Autodesk Inventor part; units mm, degrees
ref_plane "YZ Plane" through (0, 0, 0) normal (1, 0, 0) x (0, 1, 0)
ref_plane "XZ Plane" through (0, 0, 0) normal (0, 1, 0) x (-1, 0, 0)
ref_plane "XY Plane" through (0, 0, 0) normal (0, 0, 1) x (1, 0, 0)
sketch "Sketch1" plane through (0, 0, 0) normal (0, 0, 1) x (1, 0, 0)
  line L0 (0, 0) -> (-45.72, 0)
  line L1 (-45.72, 0) -> (-45.72, 20.32)
  line L2 (-45.72, 20.32) -> (0, 20.32)
  line L3 (0, 20.32) -> (0, 0)
  dimension "d0" = 45.72
  dimension "d1" = 20.32
extrude "Extrusion1" add sketch "Sketch1" along normal blind 4.826
sketch "Sketch2" plane through (-45.72, 0, 0) normal (0, -1, 0) x (1, 0, 0)
  line L0 (45.72, 0) -> (45.72, 4.826)
  line L1 (0, 0) -> (0, 4.826)
  line L2 (0, 0) -> (45.72, 0)
  line L3 (0, 4.826) -> (45.72, 4.826)
  line L4 (45.72, 0) -> (45.72, -28.194)
  line L5 (45.72, 4.826) -> (45.72, 20.066)
  line L6 (45.72, 20.066) -> (0, 20.066)
  line L7 (0, 20.066) -> (0, 4.826)
  line L8 (0, 0) -> (0, -28.194)
  line L9 (0, -28.194) -> (45.72, -28.194)
  line L10 (45.72, 0) -> (45.72, 4.826)
  line L11 (0, 4.826) -> (0, 0)
  dimension "d4" = 28.194
  dimension "d5" = 15.24
extrude "Extrusion2" add sketch "Sketch2" along normal blind 4.826
sketch "Sketch3" plane through (-45.72, 0, 0) normal (0, 1, 0) x (1, 0, 0)
  line L0 (45.72, 0) -> (0, 0)
  line L1 (45.72, 28.194) -> (45.72, 0)
  line L2 (0, 28.194) -> (45.72, 28.194)
  line L3 (0, 0) -> (0, 28.194)
  line L4 (22.86, 0) -> (22.86, 9.144) construction
  line L5 (22.86, 9.144) -> (45.72, 9.144)
  line L6 (22.86, 9.144) -> (0, 9.144)
  line L7 (45.72, 9.144) -> (45.72, 12.954)
  line L8 (45.72, 28.194) -> (45.72, -20.066)
  line L9 (45.72, 12.954) -> (0, 12.954)
  line L10 (0, 12.954) -> (0, 9.144)
  dimension "d8" = 9.144
  dimension "d9" = 3.81
extrude "Extrusion3" add sketch "Sketch3" along normal blind 20.32 contours L5 L6 L3 L9 L1
sketch "Sketch4" plane through (0, 0, -12.954) normal (0, 0, -1) x (-1, 0, 0)
  line L0 (0, 0) -> (0, 20.32)
  line L1 (0, 20.32) -> (45.72, 20.32)
  line L2 (45.72, 0) -> (45.72, 20.32)
  line L3 (45.72, 0) -> (0, 0)
  line L4 (22.86, 20.32) -> (22.86, 13.97) construction
  line L5 (22.86, 13.97) -> (30.48, 13.97) construction
  circle A0 centre (30.48, 13.97) radius 2.413
  circle A1 centre (15.24, 13.97) radius 2.413
  dimension "d12" = 6.35
  dimension "d13" = 7.62
  dimension "d14" = 4.826
extrude "Extrusion4" cut sketch "Sketch4" against normal through all contours A0 | A1
sketch "Sketch5" plane through (-45.72, 0, 0) normal (0, 1, 0) x (1, 0, 0)
  line L0 (45.72, 12.954) -> (0, 12.954)
  line L1 (0, 28.194) -> (45.72, 28.194)
  line L2 (45.72, 28.194) -> (45.72, 12.954) construction
  line L3 (0, 12.954) -> (0, 28.194)
  line L4 (45.72, 28.194) -> (45.72, -20.066)
  line L5 (45.72, 28.194) -> (45.72, 12.954) construction
  line L6 (45.72, 20.574) -> (0, 20.574) construction
  line L7 (22.86, 12.954) -> (22.86, 20.574) construction
  line L8 (22.86, 20.574) -> (13.97, 20.574) construction
  line L9 (22.86, 20.574) -> (31.75, 20.574) construction
  circle A0 centre (31.75, 20.574) radius 2.413
  circle A1 centre (13.97, 20.574) radius 2.413
  line L10 (45.72, 4.064) -> (0, 4.572) construction
  line L11 (0, 0) -> (0, 9.144)
  circle A2 centre (31.3866, -12.1315) radius 2.413
  circle A3 centre (13.611, -11.7365) radius 2.413
  point P0 (45.72, 0)
  dimension "d17" = 8.89
  dimension "d18" = 8.89
  dimension "d19" = 4.826
  dimension "d20" = 4.826
extrude "Extrusion5" cut sketch "Sketch5" against normal through all contours A0 | A1 | A2 | A3
properties part number "arm_to_tower_adapter"
Geometry check sheet. Reference: the model listing, model coordinates, mm. A direction names the side the tool comes from. Coordinates: 2 decimals unless noted, no trailing zeros. Order: outer loops, then holes, each group sorted by start corner. A loop starts at its lowest first (then second) coordinate and runs counter-clockwise, first axis right, second up. Notation, with made-up numbers: (-22, 83.5) -> (-7, 83.5) arc R18 cw to (-7, 92.5) -> close; hole circle Ø3 at (42.25, 27). An arc over 180 degrees is marked (long way). Use a Markdown table: item, result. Add a question column.
1. Cross-section at A-A (y = 1.75). Enter the section's corners in (x, z), and give its area (3 significant figures).
2. Set-up check for faces 4 (the face through (-23, 0, 13)), 5 (the face through (-23, 0, -20)), 6 (the face through (-12.83, 14.08, -11.08)), 7 (the face through (-23, -2, -28.194)), 8 (the face through (-23, 10, 0)): record each of +Z, -Z, +X, -X, +Y, -Y from which the full face is reachable in a straight line by a thin tool's end or side.
3. Cross-section at B-B (x = -31.75). Enter the section's corners in (y, z).
4. Cross-section at D-D (z = -10). Enter the section's corners in (x, y).
5. Cross-section at C-C (y = 13.97). Enter the section's corners in (x, z).
6. Go/stop test with flat-tipped pins: pin 1 Ø5 at (x, z) = (-26, -20.5) entering from +Y; pin 2 Ø10 at (x, y) = (-12.5, 12) entering from +Z; pin 3 Ø5.5 at (x, y) = (-15.24, 13.97) entering from -Z. Record where each tip stops, or that it passes through.
7. Material ranges on L1, parallel to Z at x = -43, y = 16.25; L2, parallel to Y at x = -15, z = 1; L3, parallel to X at y = 15, z = 2.5, recorded low to high.
8. Mould release check, pull along X, two halves, no side actions. Record for faces 1 (the face through (-23, 20.32, -11)), 2 (the face through (-14.856, -2.379, 14.487)), 3 (the face through (0, -0.5, -4.4)): pulls with the +X half, pulls with the -X half, needs draft (parallel to the pull), parting line crosses it, or undercut.
Filled sheet:
| question | item | result |
|---|---|---|
| 1 | outline | (-45.72, -12.95) -> (0, -12.95) -> (0, -9.14) -> (-45.72, -9.14) -> close; (-45.72, 0) -> (0, 0) -> (0, 4.83) -> (-45.72, 4.83) -> close |
| 1 | area | 395 mm2 |
| 2 | face 4 | +Z, +X, -X, +Y |
| 2 | face 5 | -Z, +X, -X, +Y |
| 2 | face 6 | +Z, -Z |
| 2 | face 7 | -Z, +X, -X, +Y, -Y |
| 2 | face 8 | +X, -X, +Y |
| 3 | outline | (-4.83, -28.19) -> (0, -28.19) -> (0, -22.99) -> (-4.83, -22.99) -> close; (-4.83, -18.16) -> (0, -18.16) -> (0, -12.95) -> (11.92, -12.95) -> (11.92, -9.14) -> (0, -9.14) -> (0, 0) -> (11.92, 0) -> (11.92, 4.83) -> (0, 4.83) -> (0, 9.35) -> (-4.83, 9.35) -> close; (-4.83, 14.12) -> (0, 14.12) -> (0, 20.07) -> (-4.83, 20.07) -> close; (16.02, -12.95) -> (20.32, -12.95) -> (20.32, -9.14) -> (16.02, -9.14) -> close; (16.02, 0) -> (20.32, 0) -> (20.32, 4.83) -> (16.02, 4.83) -> close |
| 4 | outline | (-45.72, -4.83) -> (0, -4.83) -> (0, 20.32) -> (-45.72, 20.32) -> close; hole circle Ø4.83 at (-30.48, 13.97); hole circle Ø4.83 at (-15.24, 13.97) |
| 5 | outline | (-45.72, -12.95) -> (-32.89, -12.95) -> (-32.89, -9.14) -> (-45.72, -9.14) -> close; (-45.72, 0) -> (-32.89, 0) -> (-32.89, 4.83) -> (-45.72, 4.83) -> close; (-28.07, -12.95) -> (-17.65, -12.95) -> (-17.65, -9.14) -> (-28.07, -9.14) -> close; (-28.07, 0) -> (-17.65, 0) -> (-17.65, 4.83) -> (-28.07, 4.83) -> close; (-12.83, -12.95) -> (0, -12.95) -> (0, -9.14) -> (-12.83, -9.14) -> close; (-12.83, 0) -> (0, 0) -> (0, 4.83) -> (-12.83, 4.83) -> close |
| 6 | pin 1 | y = 0 |
| 6 | pin 2 | z = 4.83 |
| 6 | pin 3 | z = -12.95 |
| 7 | L1 | -12.95 to -9.14, 0 to 4.83 |
| 7 | L2 | -4.83 to 11.57, 16.37 to 20.32 |
| 7 | L3 | -45.72 to -32.66, -28.3 to -17.42, -13.06 to 0 |
| 8 | face 1 | needs draft |
| 8 | face 2 | undercut |
| 8 | face 3 | pulls with the +X half |
